Geometry: final body of the model. Coordinates: model frame, mm. Coordinates: 2 decimals unless noted, no trailing zeros. Order: outer loops, then holes, each group sorted by start corner. A loop starts at its lowest first (then second) coordinate and runs counter-clockwise, first axis right, second up. Notation, with made-up numbers: (7, 3) - (60, 3) arc R28 cw to (60, 42) - close; hole circle Ø6 at (86, 82). An arc over 180 degrees is marked (long way). Use a Markdown table: item, result. Add a question column.
```python
from build123d import *

# Parameters (mm, degrees)
ESTRUSIONE_ESTRUSIONE1_DEPTH = 5
SCHIZZO2_R                   = 4
SCHIZZO2_R_2                 = 2
SCHIZZO2_R_3                 = 9.75
TAGLIO_ESTRUSIONE1_DEPTH     = 6


with BuildPart() as part:
    # Schizzo3 → Estrusione-Estrusione1 (new body)
    with BuildSketch(Plane(origin=(0, 0, 0), x_dir=(0, 0, -1), z_dir=(1, 0, 0))):
        with BuildLine():
            Line((40.160183768, 61.647051924), (40.160183768, 100.394835388))
            Line((40.160183768, 100.394835388), (12.334616938, 111.608123513))
            ThreePointArc((12.334616938, 111.608123513), (-5.305430843, 113.570729245), (-21.410737295, 106.111358555))
            Line((-21.410737295, 106.111358555), (-44.239245072, 86.647051924))
            Line((-44.239245072, 86.647051924), (-44.239245072, 61.647051924))
            Line((-44.239245072, 61.647051924), (40.160183768, 61.647051924))
        make_face()
    extrude(amount=ESTRUSIONE_ESTRUSIONE1_DEPTH)

    # Schizzo2 → Taglio-Estrusione1 (cut, through all)
    with BuildSketch(Plane(origin=(0, 0, 0), x_dir=(0, 0, -1), z_dir=(1, 0, 0))):
        with Locations((-95, 0)):
            Circle(SCHIZZO2_R)
        with Locations((201, 0)):
            Circle(SCHIZZO2_R)
        with Locations((12.990381057, 73.5)):
            Circle(SCHIZZO2_R_2)
        with Locations((-12.990381057, 73.5)):
            Circle(SCHIZZO2_R_2)
        with Locations((0, 96)):
            Circle(SCHIZZO2_R_2)
        with Locations((0, 81)):
            Circle(SCHIZZO2_R_3)
    extrude(amount=TAGLIO_ESTRUSIONE1_DEPTH, mode=Mode.SUBTRACT)


solid = part.part
```
1) Section A-A (y = 81). Return loops of the section in (x, z), then the cut area to 3 significant figures.
2) Ray query, line 1 along Y through (x, z) = (3.45, 0); line 2 along Z through (x, y) = (1.4, 73.5); line 3 along Z through (x, y) = (3.6, 81). Return the intervals inside material, ascending.
3) Draft query along Z for faces 1 (the face through (2, 98, 0)), 2 (the face through (2.46, 113.61, 5.06)), 3 (the face through (0, 94, 3)). Return one class per face: pulls with the +Z half, pulls with the -Z half, needs draft (parallel to the pull), parting line crosses it, or undercut.
4) Section D-D (z = -14). Return loops of the section in (x, y), then the cut area to 3 significant figures.
5) Section B-B (x = 2.6). Return loops of the section in (y, z).
6) Section C-C (z = 0). Return loops of the section in (x, y), then the cut area to 3 significant figures.
7) Pin query (flat end, axial travel): pin 1 (3 mm diameter, centred on y = 96, z = 0, fed in from -X); pin 2 (1.5 mm diameter, centred on x = 3, z = -20, fed in from +Y); pin 3 (6.5 mm diameter, centred on y = 73.5, z = 12.99, fed in from -X); pin 4 (1.5 mm diameter, centred on x = 3, y = 101, fed in from +Z). Return the tip coordinate at first contact, or that it passes through.
Values follow:
| question | item | result |
|---|---|---|
| 1 | outline | (0, -40.16) - (5, -40.16) - (5, -9.75) - (0, -9.75) - close; (0, 9.75) - (5, 9.75) - (5, 44.24) - (0, 44.24) - close |
| 1 | area | 324 mm² |
| 2 | line 1 | y = 61.65 to 71.25, 90.75 to 94, 98 to 114 |
| 2 | line 2 | z = -40.16 to -14.99, -10.99 to -6.23, 6.23 to 10.99, 14.99 to 44.24 |
| 2 | line 3 | z = -40.16 to -9.75, 9.75 to 44.24 |
| 3 | face 1 | undercut |
| 3 | face 2 | parting line crosses it |
| 3 | face 3 | needs draft |
| 4 | outline | (0, 61.65) - (5, 61.65) - (5, 71.77) - (0, 71.77) - close; (0, 75.23) - (5, 75.23) - (5, 110.94) - (0, 110.94) - close |
| 4 | area | 229 mm² |
| 5 | outline | (61.65, -40.16) - (100.39, -40.16) - (111.61, -12.33) arc R33 ccw to (106.11, 21.41) - (86.65, 44.24) - (61.65, 44.24) - close; hole circle Ø19.5 at (81, 0); hole circle Ø4 at (73.5, -12.99); hole circle Ø4 at (73.5, 12.99); hole circle Ø4 at (96, 0) |
| 6 | outline | (0, 61.65) - (5, 61.65) - (5, 71.25) - (0, 71.25) - close; (0, 90.75) - (5, 90.75) - (5, 94) - (0, 94) - close; (0, 98) - (5, 98) - (5, 114) - (0, 114) - close |
| 6 | area | 144 mm² |
| 7 | pin 1 | passes through |
| 7 | pin 2 | stops at y = 108.82 |
| 7 | pin 3 | stops at x = 0 |
| 7 | pin 4 | stops at z = 28.29 |
